Here's how the part is built. I have some questions about the finished solid (model axes, mm). Face numbers are marked on the shaded views. A direction names the side the tool comes from. Round coordinates to 2 decimals unless told otherwise and drop trailing zeros. Order: outer loops, then holes, each group sorted by start corner. A loop starts at its lowest first (then second) coordinate and runs counter-clockwise, first axis right, second up. Notation, with made-up numbers: (77.5, 85) -> (82.5, 85) arc R35 ccw to (82.5, 120) -> close; hole circle Ø6 at (29.5, 11.5). An arc over 180 degrees is marked (long way). Use a Markdown table: item, result. Add a question column.
(1) I want a section at A-A, the plane z = 0. Please give me the cut outline in (x, y) (3 decimals), then the cut area to 3 significant figures.
(2) If I drill on probe 1 along Y at (x, z) = (6, -1.25); probe 2 along Z at (x, y) = (8.5, -3.75) (3 decimals); probe 3 along Y at (x, z) = (-9.5, 1.25), over which ranges is the centre line in solid material (lowest first)?
(3) On a 3-axis mill with a long thin cutter (end or side, diameter ignored), from which of +Z, -Z, +X, -X, +Y, -Y can I reach the whole of each face in a straight line? I mean the marked faces 1, 2 and 3. Say none if no direction works.
(4) I want a section at D-D, the plane y = -4.5. Please give me the cut outline in (x, z) (3 decimals), then the cut area to 3 significant figures.
(5) I'm going to push flat-ended pins straight in: P1, Ø10, axis at x = 7.5, y = 4.5, coming from the +Z side (3 decimals); P2, Ø1, axis at x = 1, y = 11.5, coming from the +Z side; P3, Ø10, axis at y = -3, z = -11, coming from the +X side. Where does each tip first touch, or does it pass through?
(6) I want a section at C-C, the plane y = 3.75. Please give me the cut outline in (x, z).
(7) I want a section at B-B, the plane x = 0. Please give me the cut outline in (y, z) (3 decimals), then the cut area to 3 significant figures.
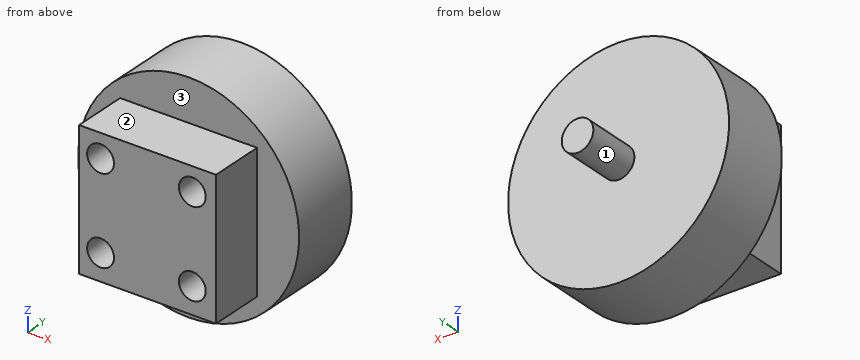
from build123d import *

# Parameters (mm, degrees)
SKETCH1_R           = 14
BOSS_EXTRUDE1_DEPTH = 9
SKETCH3_W           = 17.35
SKETCH3_H           = 17.35
BOSS_EXTRUDE2_DEPTH = 7
SKETCH4_R           = 1.7
CUT_EXTRUDE1_DEPTH  = 7
SKETCH5_R           = 2
BOSS_EXTRUDE3_DEPTH = 7


with BuildPart() as part:
    # Sketch1 → Boss-Extrude1 (new body)
    with BuildSketch(Plane(origin=(0, 0, 0), x_dir=(1, 0, 0), z_dir=(0, 1, 0))):
        with Locations(Location((0, 0, 0), (0, 0, 270))):
            Circle(SKETCH1_R)
    extrude(amount=BOSS_EXTRUDE1_DEPTH)

    # Sketch3 → Boss-Extrude2 (add)
    with BuildSketch(Plane.XZ):
        Rectangle(SKETCH3_W, SKETCH3_H)
    extrude(amount=BOSS_EXTRUDE2_DEPTH)

    # Sketch4 → Cut-Extrude1 (cut)
    with BuildSketch(Plane.XZ.offset(7)):
        with Locations(Location((-5.952043792, 5.675, 0), (0, 0, 270))):
            Circle(SKETCH4_R)
        with Locations(Location((-5.952043792, -5.316444521, 0), (0, 0, 270))):
            Circle(SKETCH4_R)
        with Locations(Location((5.675, -5.316444521, 0), (0, 0, 270))):
            Circle(SKETCH4_R)
        with Locations(Location((5.675, 5.675, 0), (0, 0, 270))):
            Circle(SKETCH4_R)
    extrude(amount=-CUT_EXTRUDE1_DEPTH, mode=Mode.SUBTRACT)

    # Sketch5 → Boss-Extrude3 (add)
    with BuildSketch(Plane(origin=(0, 9, 0), x_dir=(1, 0, 0), z_dir=(0, 1, 0))):
        with Locations(Location((0, 0, 0), (0, 0, 270))):
            Circle(SKETCH5_R)
    extrude(amount=BOSS_EXTRUDE3_DEPTH)


solid = part.part
Taken from the geometry:
| question | item | result |
|---|---|---|
| 1 | outline | (-14, 0) -> (-8.675, 0) -> (-8.675, -7) -> (8.675, -7) -> (8.675, 0) -> (14, 0) -> (14, 9) -> (2, 9) -> (2, 16) -> (-2, 16) -> (-2, 9) -> (-14, 9) -> close |
| 1 | area | 401 mm2 |
| 2 | probe 1 | y = -7 to 9 |
| 2 | probe 2 | z = -8.675 to 8.675 |
| 2 | probe 3 | y = 0 to 9 |
| 3 | face 1 | +Y |
| 3 | face 2 | +Z, +X, -X, -Y |
| 3 | face 3 | -Y |
| 4 | outline | (-8.675, -8.675) -> (8.675, -8.675) -> (8.675, 8.675) -> (-8.675, 8.675) -> close; hole circle Ø3.4 at (-5.952, -5.316); hole circle Ø3.4 at (-5.952, 5.675); hole circle Ø3.4 at (5.675, -5.316); hole circle Ø3.4 at (5.675, 5.675) |
| 4 | area | 265 mm2 |
| 5 | P1 | stops at z = 13.775 |
| 5 | P2 | stops at z = 1.94 |
| 5 | P3 | stops at x = 12.12 |
| 6 | outline | circle Ø28 at (0, 0) |
| 7 | outline | (-7, -8.675) -> (0, -8.675) -> (0, -14) -> (9, -14) -> (9, -2) -> (16, -2) -> (16, 2) -> (9, 2) -> (9, 14) -> (0, 14) -> (0, 8.675) -> (-7, 8.675) -> close |
| 7 | area | 401 mm2 |
